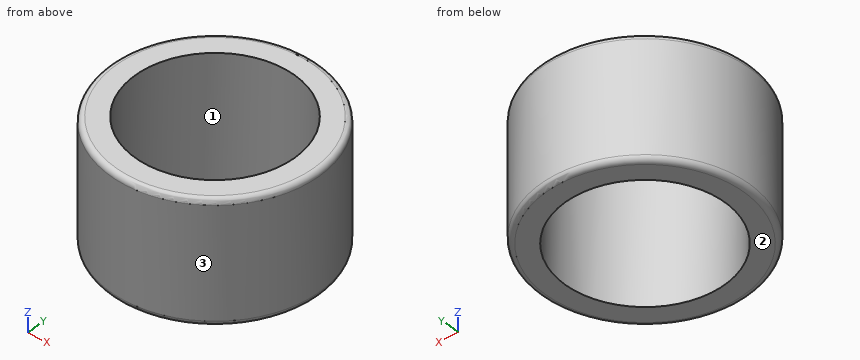
from build123d import *

# Parameters (mm, degrees)
CYLINDER041_R     = 10.5
CYLINDER041_DEPTH = 20
CYLINDER040_R     = 13.75
CYLINDER040_DEPTH = 16
FILLET013_R       = 0.7


with BuildPart() as cylinder041:
    # Cylinder041 → Cylinder041 (new body)
    with BuildSketch(Plane.XY.offset(-1)):
        Circle(CYLINDER041_R)
    extrude(amount=CYLINDER041_DEPTH)


with BuildPart() as obj1:
    # Cylinder040 → Cylinder040 (new body)
    with BuildSketch(Plane.XY):
        Circle(CYLINDER040_R)
    extrude(amount=CYLINDER040_DEPTH)

    # Cut027: cut Cylinder041
    add(cylinder041.part, mode=Mode.SUBTRACT)

    # Fillet013
    fillet013_edges = [obj1.edges().sort_by_distance(p)[0] for p in [
        (-13.75, 0, 16),
        (-13.75, 0, 0),
    ]]
    fillet(fillet013_edges, radius=FILLET013_R)


solid = obj1.part
For this review, take the finished solid that the model builds, in its own axes (mm). Face numbers are marked on the shaded views. Coordinates: 2 decimals unless noted, no trailing zeros. Loops run counter-clockwise (first coordinate to the right, second up) from the corner with the lowest first, then second, coordinate; pieces in that order, holes last. Notation, with made-up numbers: (43, 46) - (101, 46) arc R9 cw to (101, 62) - close; hole circle Ø7 at (-39.5, 11). An arc over 180 degrees is marked (long way). Use a Markdown table: item, result. Add a question column.
Item 1: We need section C-C (z = 7.75). Give the boundary of the cut face in (x, y), and give its area (3 significant figures).
Item 2: Insertion check: pin 1 Ø12.5 at (x, y) = (0, 0) entering from -Z; pin 2 Ø4 at (x, z) = (7, 14) entering from -Y; pin 3 Ø6 at (y, z) = (9.5, 12) entering from -X; pin 4 Ø1 at (x, z) = (10, 4.5) entering from +Y. Each pin has a flat end and moves straight along its axis. Give the tip position at first contact, or say it passes through.
Item 3: We need section A-A (y = 0). Give the boundary of the cut face in (x, z), and give its area (3 significant figures).
Item 4: Mouldability with a two-part tool opening along Y and no side actions: class the marked faces 1, 2 and 3 as pulls with the +Y half, pulls with the -Y half, needs draft (parallel to the pull), parting line crosses it, or undercut.
Item 5: For line 1 (Y direction, x = 0, z = 13); line 2 (Y direction, x = -9.5, z = 10.5); line 3 (X direction, y = 3.5, z = 6.5), list the stretches that pass through material, from the lowest coordinate up.
Results list:
| question | item | result |
|---|---|---|
| 1 | outline | circle Ø27.5 at (0, 0); hole circle Ø21 at (0, 0) |
| 1 | area | 248 mm^2 |
| 2 | pin 1 | passes through |
| 2 | pin 2 | stops at y = -12.81 |
| 2 | pin 3 | stops at x = -12.12 |
| 2 | pin 4 | stops at y = 9.94 |
| 3 | outline | (-13.75, 0.7) arc R0.7 ccw to (-13.05, 0) - (-10.5, 0) - (-10.5, 16) - (-13.05, 16) arc R0.7 ccw to (-13.75, 15.3) - close; (10.5, 0) - (13.05, 0) arc R0.7 ccw to (13.75, 0.7) - (13.75, 15.3) arc R0.7 ccw to (13.05, 16) - (10.5, 16) - close |
| 3 | area | 104 mm^2 |
| 4 | face 1 | undercut |
| 4 | face 2 | needs draft |
| 4 | face 3 | parting line crosses it |
| 5 | line 1 | y = -13.75 to -10.5, 10.5 to 13.75 |
| 5 | line 2 | y = -9.94 to -4.47, 4.47 to 9.94 |
| 5 | line 3 | x = -13.3 to -9.9, 9.9 to 13.3 |
